For this review, take the finished solid that the model builds, in its own axes (mm). Coordinates: 2 decimals unless noted, no trailing zeros. Order: outer loops, then holes, each group sorted by start corner. A loop starts at its lowest first (then second) coordinate and runs counter-clockwise, first axis right, second up. Notation, with made-up numbers: M 61.25,77 L 97.25,77 A10 cw 97.25,85 Z; hole C -11,-31 d3. An arc over 180 degrees is marked long. Use one line per item in the form item = value. Start each with the question number.
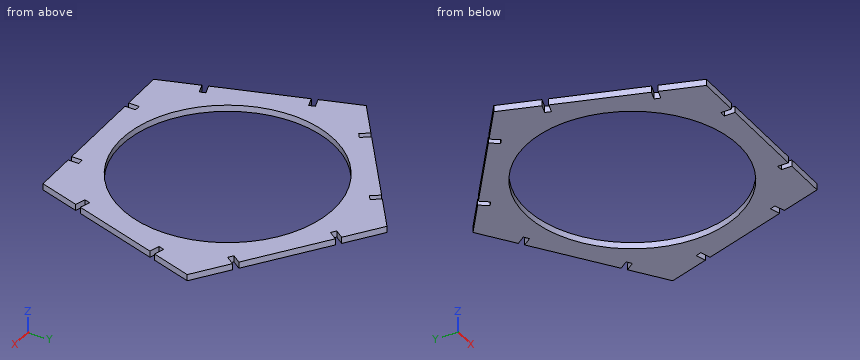
```python
from build123d import *

# Parameters (mm, degrees)
F0_R     = 50
F1_DEPTH = 3


with BuildPart() as f1:
    # F0 (on Top) → F1 (new body)
    with BuildSketch(Plane.XY):
        Polygon((16.186687, 63.152809), (0, 74.899773), (-16.173988, 63.13533), (-13.232877, 59.091833), (-15.497236, 57.444811), (-18.438346, 61.488308), (-52.862891, 36.448993), (-49.92178, 32.405496), (-52.186139, 30.758474), (-55.127249, 34.801971), (-71.301237, 23.037529), (-65.110625, 4.019739), (-60.356177, 5.567392), (-59.489492, 2.904902), (-64.243939, 1.357249), (-51.067905, -39.120012), (-46.313457, -37.572359), (-45.446772, -40.23485), (-50.201219, -41.782503), (-44.010606, -60.800292), (-24.010609, -60.78949), (-24.01331, -55.789491), (-21.21331, -55.787978), (-21.21061, -60.787978), (21.357172, -60.764986), (21.354471, -55.764987), (24.154471, -55.763475), (24.157172, -60.763474), (44.157169, -60.752671), (50.327234, -41.728206), (45.571118, -40.185689), (46.434927, -37.522264), (51.191043, -39.064781), (64.323345, 1.42669), (59.567228, 2.969207), (60.431037, 5.632632), (65.187154, 4.090116), (71.357219, 23.114581), (55.170532, 34.861545), (52.233791, 30.814873), (49.967655, 32.459448), (52.904396, 36.50612), (18.452823, 61.508234), (15.516082, 57.461562), (13.249946, 59.106137), align=None)
        Circle(F0_R, mode=Mode.SUBTRACT)
    extrude(amount=F1_DEPTH)


solid = f1.part
```
1. To check wall thickness, follow line 1 (Y direction, x = 0, z = 1.35); line 2 (Y direction, x = -32.5, z = 2.3); line 3 (X direction, y = -6, z = 0.65). State the ranges of each line that lie inside material, in increasing order.
2. Consider section B-B, the plane y = -19. Write out the cut boundary in (x, z).
3. For pin 1 Ø1 at (x, z) = (-14.5, 0.5) entering from -Y, flat-tipped, find the tip position at first contact; note if it passes through.
4. Consider section A-A, the plane x = -36. Write out the cut boundary in (y, z), plus the area to 3 significant figures.
Answers follow:
q1.line_1 = -60.78 to -50, 50 to 74.9
q1.line_2 = -60.79 to -38, 38 to 51.26
q1.line_3 = -61.85 to -49.64, 49.64 to 61.91
q2.outline = M -57.62,0 L -46.25,0 L -46.25,3 L -57.62,3 Z; M 46.25,0 L 57.7,0 L 57.7,3 L 46.25,3 Z
q3.pin_1 = -60.78
q4.outline = M -60.8,0 L -34.7,0 L -34.7,3 L -60.8,3 Z; M 34.7,0 L 48.71,0 L 48.71,3 L 34.7,3 Z
q4.area = 120 mm²
